from build123d import *

# Parameters (mm, degrees)
SKETCH1_R           = 64.9605
BOSS_EXTRUDE1_DEPTH = 15.24
CUT_EXTRUDE1_DEPTH  = 30.48
FILLET1_R           = 6.35


with BuildPart() as part:
    # Sketch1 → Boss-Extrude1 (new, symmetric)
    with BuildSketch(Plane(origin=(0, 0, 0), x_dir=(1, 0, 0), z_dir=(0, 1, 0))):
        Circle(SKETCH1_R)
    extrude(amount=BOSS_EXTRUDE1_DEPTH, both=True)

    # Sketch2 → Cut-Extrude1 (cut)
    with BuildSketch(Plane(origin=(0, 15.24, 0), x_dir=(1, 0, 0), z_dir=(0, 1, 0))):
        Polygon((7.332348419, 8.887e-06), (3.666166513, 6.350004444), (-3.666181906, 6.349995556), (-7.332348419, -8.887e-06), (-3.666166513, -6.350004444), (3.666181906, -6.349995556), align=None)
    extrude(amount=-CUT_EXTRUDE1_DEPTH, mode=Mode.SUBTRACT)

    # Fillet1
    fillet1_edges = [part.edges().sort_by_distance(p)[0] for p in [
        (-64.9605, -15.24, 0),
        (-64.9605, 15.24, 0),
    ]]
    fillet(fillet1_edges, radius=FILLET1_R)


solid = part.part
Read the model definition and answer for the solid it produces. Units are mm, in the model's axes. A direction names the side the tool comes from. Round coordinates to 2 decimals unless told otherwise and drop trailing zeros. Write each loop counter-clockwise with the first axis right and the second up, starting at its lowest first coordinate (ties: lowest second). Pieces come first, ordered by that corner, then holes. Notation, with made-up numbers: (70.25, 6) - (78.25, 6) arc R22 cw to (78.25, 18) - close; hole circle Ø5 at (59, 63.25). An arc over 180 degrees is marked (long way). One line per question, with ' | ' between items. Start each with the question number.
1. Find the intervals of material crossed by probe 1 along X at (y, z) = (-1, -3); probe 2 along X at (y, z) = (-6, -1) (3 decimals); probe 3 along Z at (x, y) = (-3.5, 6), in increasing order. Write a range as [from, to].
2. Section A-A (x = 0) is taken. Determine the outline of the cut face in (y, z).
3. Section B-B (y = -3) is taken. Determine the outline of the cut face in (x, z).
4. For faces 1 (the face through (12, -15.24, -1)), 2 (the face through (-5.525, 0.213, 3.131)), determine the directions among +Z, -Z, +X, -X, +Y, -Y from which every point of the face is accessible in a straight line to the end or side of a thin tool.
5. For a pull along X with two mould halves and no side action, classify faces 3 (the face through (5.474, 0.213, 3.219)), 4 (the face through (12, 15.24, -1)), 5 (the face through (-8.5, 0.1, -64.4)) as +X half, -X half, draft (parallel to the pull), parting line (faces both ways), or undercut.
6. Each of these flat-tipped pins is pushed along its axis until it touches: pin 1 (4 mm diameter, centred on x = 47, z = 47, fed in from -Y); pin 2 (4 mm diameter, centred on x = -30, y = -3, fed in from +Z); pin 3 (1 mm diameter, centred on x = -37.5, y = 7, fed in from +Z). Where does it stop, or does it pass through?
7. Section C-C (y = 10.5) is taken. Determine the outline of the cut face in (x, z).
Filled in:
1) probe 1: [-64.89, -5.6], [5.6, 64.89] | probe 2: [-64.953, -6.755], [6.755, 64.953] | probe 3: [-64.87, -6.35], [6.35, 64.87]
2) outline: (-15.24, -58.61) arc R6.35 ccw to (-8.89, -64.96) - (8.89, -64.96) arc R6.35 ccw to (15.24, -58.61) - (15.24, -6.35) - (-15.24, -6.35) - close; (-15.24, 6.35) - (15.24, 6.35) - (15.24, 58.61) arc R6.35 ccw to (8.89, 64.96) - (-8.89, 64.96) arc R6.35 ccw to (-15.24, 58.61) - close
3) outline: circle Ø129.92 at (0, 0); hole (-7.33, 0) - (-3.67, -6.35) - (3.67, -6.35) - (7.33, 0) - (3.67, 6.35) - (-3.67, 6.35) - close
4) face 1: +Z, -Z, +X, -X, -Y | face 2: +Y, -Y
5) face 3: undercut | face 4: draft | face 5: parting line
6) pin 1: y = -11.34 | pin 2: z = 58.62 | pin 3: z = 53.39
7) outline: circle Ø129.51 at (0, 0); hole (-7.33, 0) - (-3.67, -6.35) - (3.67, -6.35) - (7.33, 0) - (3.67, 6.35) - (-3.67, 6.35) - close
